The listing builds one solid part. Answer for the finished solid, in the listing's coordinates (mm). Face numbers are marked on the shaded views. Coordinates: 2 decimals unless noted, no trailing zeros. Write each loop counter-clockwise with the first axis right and the second up, starting at its lowest first coordinate (ties: lowest second). Pieces come first, ordered by that corner, then holes.
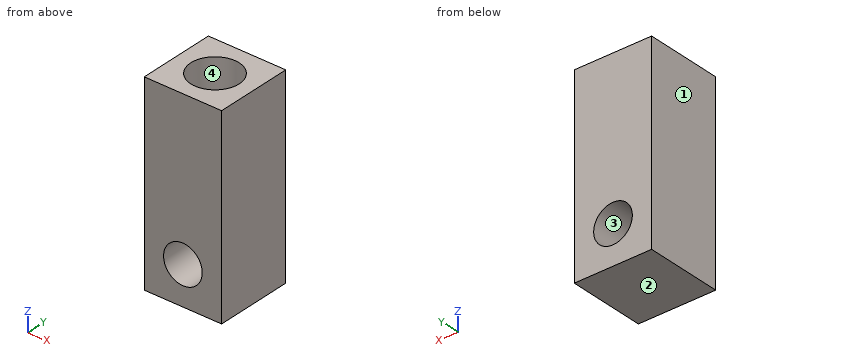
from build123d import *

# Parameters (mm, degrees)
F0_W     = 5.08
F0_H     = 5.08
F1_DEPTH = 12.7
F2_R     = 1.27
F3_DEPTH = 5.081
F4_R     = 1.5875
F5_DEPTH = 7.62


with BuildPart() as f1:
    # F0 (on Top) → F1 (new body)
    with BuildSketch(Plane.XY):
        with Locations((-2.54, 2.54)):
            Rectangle(F0_W, F0_H)
    extrude(amount=F1_DEPTH)

    # F2 (on face) → F3 (cut, through all)
    with BuildSketch(Plane.XZ):
        with Locations((-2.543417, 2.54)):
            Circle(F2_R)
    extrude(amount=-F3_DEPTH, mode=Mode.SUBTRACT)

    # F4 (on face) → F5 (cut)
    with BuildSketch(Plane.XY.offset(12.7)):
        with Locations((-2.54, 2.54)):
            Circle(F4_R)
    extrude(amount=-F5_DEPTH, mode=Mode.SUBTRACT)


solid = f1.part
Q1. The part is cut by section B-B, the plane x = -2.54. Write down the section's boundary in (y, z), then the cut area to 3 significant figures.
Answers below:
outline: (0, 0) - (5.08, 0) - (5.08, 1.27) - (0, 1.27) - close; (0, 3.81) - (5.08, 3.81) - (5.08, 12.7) - (4.13, 12.7) - (4.13, 5.08) - (0.95, 5.08) - (0.95, 12.7) - (0, 12.7) - close
area: 27.4 mm2
Q2. Determine the mould class of the marked faces 1, 2, 3 and 4 for opening direction X: released by +X, released by -X, zero draft, split by the parting line, or undercut.
Answers below:
face 1: released by -X
face 2: zero draft
face 3: undercut
face 4: undercut
Q3. Find the intervals of material crossed by probe 1 along Y at (x, z) = (-2.54, 8.75); probe 2 along X at (y, z) = (1, 1.75); probe 3 along Z at (x, y) = (-1.65, 0.3), in increasing order.
Answers below:
probe 1: y = 0 to 0.95, 4.13 to 5.08
probe 2: x = -5.08 to -3.54, -1.55 to 0
probe 3: z = 0 to 1.64, 3.44 to 12.7
Q4. The part is cut by section D-D, the plane z = 8.5. Write down the section's boundary in (x, y) (1 decimal), then the cut area to 3 significant figures.
Answers below:
outline: (-5.1, 0) - (0, 0) - (0, 5.1) - (-5.1, 5.1) - close; hole circle Ø3.2 at (-2.5, 2.5)
area: 17.9 mm2
Q5. The part is cut by section C-C, the plane y = 0.55. Write down the section's boundary in (x, z), then the cut area to 3 significant figures.
Answers below:
outline: (-5.08, 0) - (0, 0) - (0, 12.7) - (-5.08, 12.7) - close; hole circle Ø2.54 at (-2.54, 2.54)
area: 59.4 mm2
Q6. The part is cut by section A-A, the plane z = 2.54. Write down the section's boundary in (x, y).
Answers below:
outline: (-5.08, 0) - (-3.81, 0) - (-3.81, 5.08) - (-5.08, 5.08) - close; (-1.27, 0) - (0, 0) - (0, 5.08) - (-1.27, 5.08) - close
